The drawing under review shows one solid part. Ordinate dimensions are in mm from its lowest x, y, z. A direction names the side the tool comes from. Coordinates: 2 decimals unless noted, no trailing zeros. Order: outer loops, then holes, each group sorted by start corner. A loop starts at its lowest first (then second) coordinate and runs counter-clockwise, first axis right, second up.
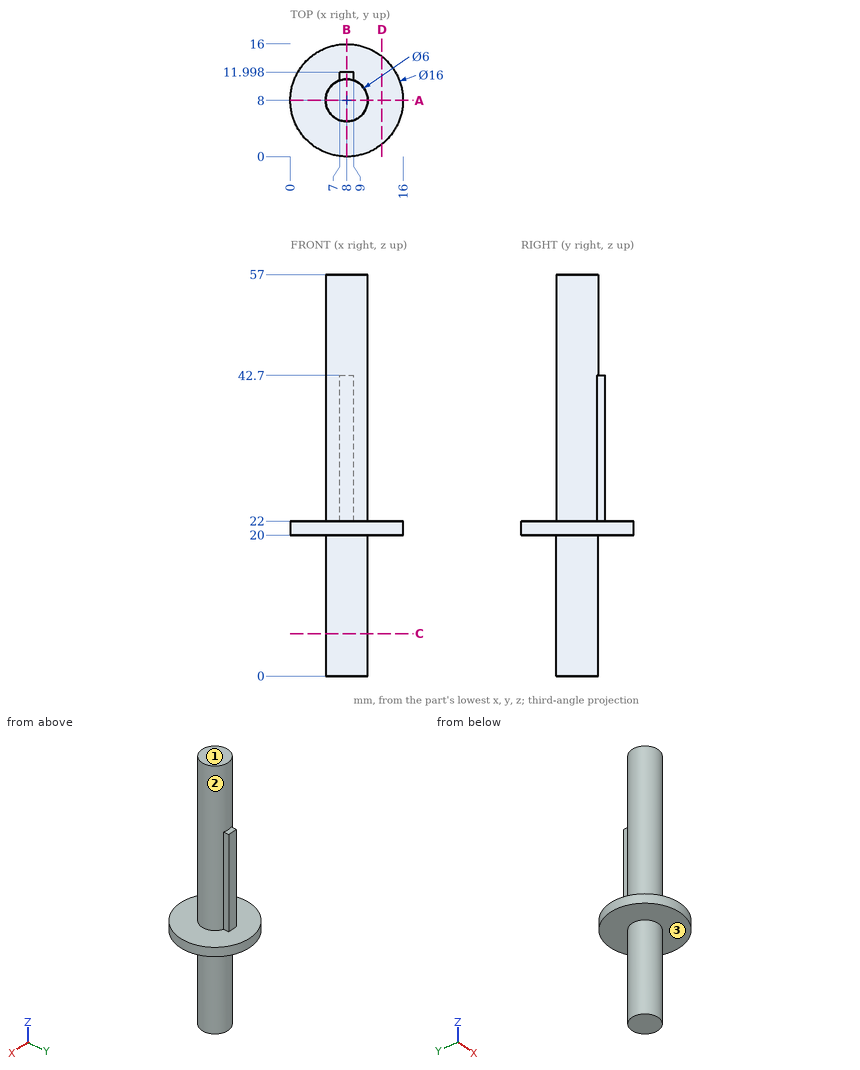
(1) We need section A-A, the plane y = 8. Write out the cut boundary in (x, z), and give its area (3 significant figures).
A:
outline: (0, 20) - (5, 20) - (5, 0) - (11, 0) - (11, 20) - (16, 20) - (16, 22) - (11, 22) - (11, 57) - (5, 57) - (5, 22) - (0, 22) - close
area: 362 mm2
(2) Wall thickness on probe 1 along Z at (x, y) = (4.75, 7); probe 2 along Z at (x, y) = (7.25, 11.75); probe 3 along X at (y, z) = (7, 54): over which ranges is each line inside the solid? List them lowest first.
A:
probe 1: z = 20 to 22
probe 2: z = 20 to 42.7
probe 3: x = 5.17 to 10.83
(3) Machinability: for the marked faces 1, 2 and 3, which of the approach directions +Z, -Z, +X, -X, +Y, -Y give a long, thin tool a straight path to every point of the face, cutting with its end or side? Answer none if there is none.
A:
face 1: +Z, +X, -X, +Y, -Y
face 2: +Z
face 3: -Z
(4) We need section B-B, the plane x = 8. Write out the cut boundary in (y, z).
A:
outline: (0, 20) - (5, 20) - (5, 0) - (11, 0) - (11, 20) - (16, 20) - (16, 22) - (12, 22) - (12, 42.7) - (11, 42.7) - (11, 57) - (5, 57) - (5, 22) - (0, 22) - close
(5) We need section C-C, the plane z = 6. Write out the cut boundary in (x, y).
A:
outline: circle Ø6 at (8, 8)
(6) For pin 1 Ø1 at (x, z) = (5.5, 26.5) entering from -Y (1 decimal); pin 2 Ø3 at (y, z) = (10.5, 51) entering from -X; pin 3 Ø3 at (x, z) = (9.5, 9.5) entering from -Y, all flat-tipped, find the tip position at first contact; note any pin that passes through.
A:
pin 1: stops at y = 5.8
pin 2: stops at x = 5.17
pin 3: stops at y = 5
(7) We need section D-D, the plane x = 13. Write out the cut boundary in (y, z) (1 decimal), and give its area (3 significant figures).
A:
outline: (1.8, 20) - (14.2, 20) - (14.2, 22) - (1.8, 22) - close
area: 25.0 mm2
